Input: part model. Units: mm. Frame: model coordinates. A direction names the side the tool comes from. Give positions to 0.01 mm unless a question says otherwise; leave off trailing zeros. Loops run counter-clockwise (first coordinate to the right, second up) from the corner with the lowest first, then second, coordinate; pieces in that order, holes last. Notation, with made-up numbers: M -25,13.5 L 23,13.5 A29 cw 23,41.5 Z; hole C 73,77 d7. An arc over 180 degrees is marked long. Answer as a JSON object with one key per item and string values. Group by question number.
1) Section query C-C on y = 16. Count the separate pieces of the cut face and the enclosed holes in it, plus the area to 3 significant figures.
2) Section query A-A on y = 39. Return loops of the section in (x, z), plus the area to 4 significant figures.
3) Access query for faces 1 (the cylindrical face through (35.473, 40.859, 1.479)), 2 (the flat face through (150, 10, 1)). Directions: +Z, -Z, +X, -X, +Y, -Y. A direction counts if a zero-diameter tool reaches every point of the face in a straight line with its end or side. Return the directions, or none.
4) Section query B-B on x = 7. Return loops of the section in (y, z), plus the area to 4 significant figures.
5) Draft query along X for faces 3 (the flat face through (0, 22, 1)), 4 (the flat face through (102.5, 20, 1.5)), 5 (the flat face through (31, 0, 1)). Return one class per face: +X half, -X half, draft (parallel to the pull), parting line (faces both ways), or undercut.
6) Ray query, L1, parallel to Y at x = 83.5, z = 0.9; L2, parallel to X at y = 36.5, z = 1.25; L3, parallel to Y at x = 145.5, z = 2.65. Return the intervals inside material, ascending.
7) First-contact query: P1, Ø0.5, axis at x = 83.5, z = 1.5, coming from the -Y side; P2, Ø1, axis at x = 65, z = 0.5, coming from the -Y side. Flat tips, straight axial feed; report the tip coordinate or a pass-through.
from build123d import *

# Parameters (mm, degrees)
F0_R     = 2.75
F1_DEPTH = 3


with BuildPart() as f1:
    # F0 (on Top) → F1 (new body)
    with BuildSketch(Plane.XY):
        with BuildLine():
            Line((0, 44), (0, 0))
            Line((0, 0), (15, 0))
            ThreePointArc((15, 0), (16.414214, 0.585786), (17, 2))
            Line((17, 2), (17, 18.5))
            Line((17, 18.5), (17, 19))
            ThreePointArc((17, 19), (17.87868, 21.12132), (20, 22))
            Line((20, 22), (20.5, 22))
            Line((20.5, 22), (21, 22))
            ThreePointArc((21, 22), (23.12132, 21.12132), (24, 19))
            Line((24, 19), (24, 18.5))
            Line((24, 18.5), (24, 2))
            ThreePointArc((24, 2), (24.585786, 0.585786), (26, 0))
            Line((26, 0), (36, 0))
            ThreePointArc((36, 0), (37.414214, 0.585786), (38, 2))
            Line((38, 2), (38, 18.5))
            Line((38, 18.5), (38, 19))
            ThreePointArc((38, 19), (38.87868, 21.12132), (41, 22))
            Line((41, 22), (41.5, 22))
            Line((41.5, 22), (42, 22))
            ThreePointArc((42, 22), (44.12132, 21.12132), (45, 19))
            Line((45, 19), (45, 18.5))
            Line((45, 18.5), (45, 2))
            ThreePointArc((45, 2), (45.585786, 0.585786), (47, 0))
            Line((47, 0), (57, 0))
            ThreePointArc((57, 0), (58.414214, 0.585786), (59, 2))
            Line((59, 2), (59, 18.5))
            Line((59, 18.5), (59, 19))
            ThreePointArc((59, 19), (59.87868, 21.12132), (62, 22))
            Line((62, 22), (62.5, 22))
            Line((62.5, 22), (63, 22))
            ThreePointArc((63, 22), (65.12132, 21.12132), (66, 19))
            Line((66, 19), (66, 18.5))
            Line((66, 18.5), (66, 2))
            ThreePointArc((66, 2), (66.585786, 0.585786), (68, 0))
            Line((68, 0), (78, 0))
            ThreePointArc((78, 0), (79.414214, 0.585786), (80, 2))
            Line((80, 2), (80, 18.5))
            Line((80, 18.5), (80, 19))
            ThreePointArc((80, 19), (80.87868, 21.12132), (83, 22))
            Line((83, 22), (83.5, 22))
            Line((83.5, 22), (84, 22))
            ThreePointArc((84, 22), (86.12132, 21.12132), (87, 19))
            Line((87, 19), (87, 18.5))
            Line((87, 18.5), (87, 2))
            ThreePointArc((87, 2), (87.585786, 0.585786), (89, 0))
            Line((89, 0), (99, 0))
            ThreePointArc((99, 0), (100.414214, 0.585786), (101, 2))
            Line((101, 2), (101, 18.5))
            Line((101, 18.5), (101, 19))
            ThreePointArc((101, 19), (101.87868, 21.12132), (104, 22))
            Line((104, 22), (104.5, 22))
            Line((104.5, 22), (105, 22))
            ThreePointArc((105, 22), (107.12132, 21.12132), (108, 19))
            Line((108, 19), (108, 18.5))
            Line((108, 18.5), (108, 2))
            ThreePointArc((108, 2), (108.585786, 0.585786), (110, 0))
            Line((110, 0), (118, 0))
            ThreePointArc((118, 0), (119.414214, 0.585786), (120, 2))
            Line((120, 2), (120, 17.5))
            Line((120, 17.5), (120, 18))
            ThreePointArc((120, 18), (121.171573, 20.828427), (124, 22))
            Line((124, 22), (124.5, 22))
            Line((124.5, 22), (125, 22))
            ThreePointArc((125, 22), (127.828427, 20.828427), (129, 18))
            Line((129, 18), (129, 17.5))
            Line((129, 17.5), (129, 2))
            ThreePointArc((129, 2), (129.585786, 0.585786), (131, 0))
            Line((131, 0), (139, 0))
            ThreePointArc((139, 0), (140.414214, 0.585786), (141, 2))
            Line((141, 2), (141, 17.5))
            Line((141, 17.5), (141, 18))
            ThreePointArc((141, 18), (142.171573, 20.828427), (145, 22))
            Line((145, 22), (145.5, 22))
            Line((145.5, 22), (146, 22))
            ThreePointArc((146, 22), (148.828427, 20.828427), (150, 18))
            Line((150, 18), (150, 17.5))
            Line((150, 17.5), (150, 2))
            ThreePointArc((150, 2), (150.585786, 0.585786), (152, 0))
            Line((152, 0), (167, 0))
            Line((167, 0), (167, 44))
            Line((167, 44), (0, 44))
        make_face()
        with Locations((7, 16)):
            Circle(F0_R, mode=Mode.SUBTRACT)
        with Locations((160, 16)):
            Circle(F0_R, mode=Mode.SUBTRACT)
        with Locations((37.5, 39)):
            Circle(F0_R, mode=Mode.SUBTRACT)
        with Locations((83.5, 39)):
            Circle(F0_R, mode=Mode.SUBTRACT)
        with Locations((129.5, 39)):
            Circle(F0_R, mode=Mode.SUBTRACT)
        with BuildLine():
            Line((17, 19), (17, 18.5))
            Line((17, 18.5), (20, 21.5))
            Line((20, 21.5), (20.5, 22))
            Line((20.5, 22), (20, 22))
            ThreePointArc((20, 22), (17.87868, 21.12132), (17, 19))
        make_face()
        with BuildLine():
            Line((21, 22), (20.5, 22))
            Line((20.5, 22), (21, 21.5))
            Line((21, 21.5), (24, 18.5))
            Line((24, 18.5), (24, 19))
            ThreePointArc((24, 19), (23.12132, 21.12132), (21, 22))
        make_face()
        Polygon((20.5, 22), (20, 21.5), (21, 21.5), align=None)
        with BuildLine():
            Line((38, 19), (38, 18.5))
            Line((38, 18.5), (41, 21.5))
            Line((41, 21.5), (41.5, 22))
            Line((41.5, 22), (41, 22))
            ThreePointArc((41, 22), (38.87868, 21.12132), (38, 19))
        make_face()
        Polygon((41.5, 22), (41, 21.5), (42, 21.5), align=None)
        with BuildLine():
            Line((42, 22), (41.5, 22))
            Line((41.5, 22), (42, 21.5))
            Line((42, 21.5), (45, 18.5))
            Line((45, 18.5), (45, 19))
            ThreePointArc((45, 19), (44.12132, 21.12132), (42, 22))
        make_face()
        with BuildLine():
            Line((80, 19), (80, 18.5))
            Line((80, 18.5), (83, 21.5))
            Line((83, 21.5), (83.5, 22))
            Line((83.5, 22), (83, 22))
            ThreePointArc((83, 22), (80.87868, 21.12132), (80, 19))
        make_face()
        Polygon((83.5, 22), (83, 21.5), (84, 21.5), align=None)
        with BuildLine():
            Line((84, 22), (83.5, 22))
            Line((83.5, 22), (84, 21.5))
            Line((84, 21.5), (87, 18.5))
            Line((87, 18.5), (87, 19))
            ThreePointArc((87, 19), (86.12132, 21.12132), (84, 22))
        make_face()
        with BuildLine():
            Line((101, 18.5), (104, 21.5))
            Line((104, 21.5), (104.5, 22))
            Line((104.5, 22), (104, 22))
            ThreePointArc((104, 22), (101.87868, 21.12132), (101, 19))
            Line((101, 19), (101, 18.5))
        make_face()
        Polygon((104, 21.5), (105, 21.5), (104.5, 22), align=None)
        with BuildLine():
            Line((105, 21.5), (108, 18.5))
            Line((108, 18.5), (108, 19))
            ThreePointArc((108, 19), (107.12132, 21.12132), (105, 22))
            Line((105, 22), (104.5, 22))
            Line((104.5, 22), (105, 21.5))
        make_face()
        with BuildLine():
            Line((124, 21.5), (124.5, 22))
            Line((124.5, 22), (124, 22))
            ThreePointArc((124, 22), (121.171573, 20.828427), (120, 18))
            Line((120, 18), (120, 17.5))
            Line((120, 17.5), (124, 21.5))
        make_face()
        Polygon((124, 21.5), (125, 21.5), (124.5, 22), align=None)
        with BuildLine():
            Line((125, 21.5), (129, 17.5))
            Line((129, 17.5), (129, 18))
            ThreePointArc((129, 18), (127.828427, 20.828427), (125, 22))
            Line((125, 22), (124.5, 22))
            Line((124.5, 22), (125, 21.5))
        make_face()
        with BuildLine():
            Line((141, 17.5), (145, 21.5))
            Line((145, 21.5), (145.5, 22))
            Line((145.5, 22), (145, 22))
            ThreePointArc((145, 22), (142.171573, 20.828427), (141, 18))
            Line((141, 18), (141, 17.5))
        make_face()
        Polygon((145, 21.5), (146, 21.5), (145.5, 22), align=None)
        with BuildLine():
            Line((146, 21.5), (150, 17.5))
            Line((150, 17.5), (150, 18))
            ThreePointArc((150, 18), (148.828427, 20.828427), (146, 22))
            Line((146, 22), (145.5, 22))
            Line((145.5, 22), (146, 21.5))
        make_face()
        with BuildLine():
            Line((59, 19), (59, 18.5))
            Line((59, 18.5), (62, 21.5))
            Line((62, 21.5), (62.5, 22))
            Line((62.5, 22), (62, 22))
            ThreePointArc((62, 22), (59.87868, 21.12132), (59, 19))
        make_face()
        Polygon((62.5, 22), (62, 21.5), (63, 21.5), align=None)
        with BuildLine():
            Line((63, 22), (62.5, 22))
            Line((62.5, 22), (63, 21.5))
            Line((63, 21.5), (66, 18.5))
            Line((66, 18.5), (66, 19))
            ThreePointArc((66, 19), (65.12132, 21.12132), (63, 22))
        make_face()
    extrude(amount=F1_DEPTH)


solid = f1.part
Output:
{
 "1": {"separate pieces": "10", "enclosed holes": "0", "area": "309 mm^2"},
 "2": {"outline": "M 0,0 L 34.75,0 L 34.75,3 L 0,3 Z; M 40.25,0 L 80.75,0 L 80.75,3 L 40.25,3 Z; M 86.25,0 L 126.75,0 L 126.75,3 L 86.25,3 Z; M 132.25,0 L 167,0 L 167,3 L 132.25,3 Z", "area": "451.5 mm^2"},
 "3": {"face 1": "+Z, -Z", "face 2": "+Z, -Z, -Y"},
 "4": {"outline": "M 0,0 L 13.25,0 L 13.25,3 L 0,3 Z; M 18.75,0 L 44,0 L 44,3 L 18.75,3 Z", "area": "115.5 mm^2"},
 "5": {"face 3": "-X half", "face 4": "undercut", "face 5": "draft"},
 "6": {"L1": "y = 21.5 to 36.25, 41.75 to 44", "L2": "x = 0 to 36.35, 38.65 to 82.35, 84.65 to 128.35, 130.65 to 167", "L3": "y = 21.5 to 44"},
 "7": {"P1": "stops at y = 21.5", "P2": "stops at y = 19"}
}
